Autodesk Inventor part; units mm, degrees
ref_plane "YZ Plane" through (0, 0, 0) normal (1, 0, 0) x (0, 1, 0)
ref_plane "XZ Plane" through (0, 0, 0) normal (0, 1, 0) x (-1, 0, 0)
ref_plane "XY Plane" through (0, 0, 0) normal (0, 0, 1) x (1, 0, 0)
sketch "스케치1" plane through (0, 0, 0) normal (0, 1, 0) x (-1, 0, 0)
  line L0 (23.5, -7) -> (-23.5, -7) construction
  line L1 (-23.5, -7) -> (-23.5, 7) construction
  line L2 (-23.5, 7) -> (23.5, 7) construction
  line L3 (23.5, 7) -> (23.5, -7) construction
  circle A0 centre (23.5, -7) radius 2.1
  circle A1 centre (-23.5, 7) radius 2.1
  circle A2 centre (0, -20) radius 2.1
  circle A3 centre (0, 20) radius 2.1
  circle A4 centre (0, 0) radius 4.5
  circle A5 centre (8, 0) radius 1.6
  circle A6 centre (0, 9.5) radius 1.6
  circle A7 centre (-8, 0) radius 1.6
  circle A8 centre (0, -9.5) radius 1.6
  line L4 (8, 0) -> (0, -9.5) construction
  line L5 (0, -9.5) -> (-8, 0) construction
  line L6 (-8, 0) -> (0, 9.5) construction
  line L7 (0, 9.5) -> (8, 0) construction
  line L8 (10, -10) -> (17, -17) construction
  line L9 (8.8686, -11.1314) -> (15.8686, -18.1314)
  line L10 (18.1314, -15.8686) -> (11.1314, -8.8686)
  arc A9 (11.1314, -8.8686) -> (8.8686, -11.1314) centre (10, -10) ccw
  arc A10 (15.8686, -18.1314) -> (18.1314, -15.8686) centre (17, -17) ccw
  line L11 (-10, -10) -> (-17, -17) construction
  line L12 (-11.1314, -8.8686) -> (-18.1314, -15.8686)
  line L13 (-15.8686, -18.1314) -> (-8.8686, -11.1314)
  arc A11 (-8.8686, -11.1314) -> (-11.1314, -8.8686) centre (-10, -10) ccw
  arc A12 (-18.1314, -15.8686) -> (-15.8686, -18.1314) centre (-17, -17) ccw
  line L14 (10, 10) -> (17, 17) construction
  line L15 (11.1314, 8.8686) -> (18.1314, 15.8686)
  line L16 (15.8686, 18.1314) -> (8.8686, 11.1314)
  arc A13 (8.8686, 11.1314) -> (11.1314, 8.8686) centre (10, 10) ccw
  arc A14 (18.1314, 15.8686) -> (15.8686, 18.1314) centre (17, 17) ccw
  line L17 (-10, 10) -> (-17, 17) construction
  line L18 (-8.8686, 11.1314) -> (-15.8686, 18.1314)
  line L19 (-18.1314, 15.8686) -> (-11.1314, 8.8686)
  arc A15 (-11.1314, 8.8686) -> (-8.8686, 11.1314) centre (-10, 10) ccw
  arc A16 (-15.8686, 18.1314) -> (-18.1314, 15.8686) centre (-17, 17) ccw
  line L20 (10, -10) -> (-10, -10) construction
  line L21 (-10, -10) -> (-10, 10) construction
  line L22 (-10, 10) -> (10, 10) construction
  line L23 (10, 10) -> (10, -10) construction
  circle A17 centre (0, 0) radius 30
  line L24 (42, 0) -> (-42, 0)
  line L25 (0, -42) -> (0, 42)
  line L26 (0, 9.5) -> (0, -9.5) construction
  line L27 (8, 0) -> (-8, 0) construction
  line L28 (28.5, -25) -> (-28.5, -25)
  line L29 (-28.5, -25) -> (-28.5, 25)
  line L30 (-28.5, 25) -> (28.5, 25)
  line L31 (28.5, 25) -> (28.5, -25)
  point P0 (13.5, -13.5)
  point P1 (-13.5, -13.5)
  point P2 (13.5, 13.5)
  point P3 (-13.5, 13.5)
  dimension "d0" = 4.2
  dimension "d1" = 40
  dimension "d2" = 47
  dimension "d3" = 14
  dimension "d4" = 3.2
  dimension "d5" = 16
  dimension "d6" = 19
  dimension "d7" = 9
  dimension "d8" = 20
  dimension "d9" = 34
  dimension "d10" = 1.6
  dimension "d11" = 60
  dimension "d18" = 5
  dimension "d19" = 5
extrude "돌출1" add sketch "스케치1" along normal blind 5 contours A2 L25 A8 A4 L24 A5 L31 A17 L28 | A2 L25 L28 A17 L29 L24 A7 A4 A8 | L28 A17 L25 | L25 A17 L28 | L31 L24 A17 | A17 L24 L29 | L24 A7 L29 A17 L30 L25 A3 A6 A4 | A4 L25 A6 A3 L30 A17 L31 L24 A5 | L24 L31 A17 | A17 L29 L24 | L30 L25 A17 | A17 L25 L30
sketch "스케치2" plane through (0, 0, 0) normal (0, -1, 0) x (1, 0, 0)
  circle A0 centre (0, 0) radius 30
  circle A1 centre (0, 0) radius 4.5
  circle A2 centre (8, 0) radius 1.6
  circle A3 centre (0, -20) radius 2.1
  circle A4 centre (0, -9.5) radius 1.6
  circle A5 centre (-8, 0) radius 1.6
  arc A6 (8.8686, 11.1314) -> (11.1314, 8.8686) centre (10, 10) ccw
  line L0 (15.8686, 18.1314) -> (8.8686, 11.1314)
  arc A7 (18.1314, 15.8686) -> (15.8686, 18.1314) centre (17, 17) ccw
  line L1 (11.1314, 8.8686) -> (18.1314, 15.8686)
  circle A8 centre (23.5, 7) radius 2.1
  arc A9 (-11.1314, 8.8686) -> (-8.8686, 11.1314) centre (-10, 10) ccw
  line L2 (-18.1314, 15.8686) -> (-11.1314, 8.8686)
  arc A10 (-15.8686, 18.1314) -> (-18.1314, 15.8686) centre (-17, 17) ccw
  line L3 (-8.8686, 11.1314) -> (-15.8686, 18.1314)
  circle A11 centre (0, 20) radius 2.1
  circle A12 centre (0, 9.5) radius 1.6
  circle A13 centre (-23.5, -7) radius 2.1
  arc A14 (-8.8686, -11.1314) -> (-11.1314, -8.8686) centre (-10, -10) ccw
  line L4 (-15.8686, -18.1314) -> (-8.8686, -11.1314)
  arc A15 (-18.1314, -15.8686) -> (-15.8686, -18.1314) centre (-17, -17) ccw
  line L5 (-11.1314, -8.8686) -> (-18.1314, -15.8686)
  arc A16 (11.1314, -8.8686) -> (8.8686, -11.1314) centre (10, -10) ccw
  line L6 (18.1314, -15.8686) -> (11.1314, -8.8686)
  arc A17 (15.8686, -18.1314) -> (18.1314, -15.8686) centre (17, -17) ccw
  line L7 (8.8686, -11.1314) -> (15.8686, -18.1314)
  circle A18 centre (0, 20) radius 5
  circle A19 centre (23.5, 7) radius 2.1
  circle A20 centre (23.5, 7) radius 5
  circle A21 centre (0, -20) radius 2.1
  circle A22 centre (0, -20) radius 5
  circle A23 centre (-23.5, -7) radius 2.1
  circle A24 centre (-23.5, -7) radius 5
  dimension "d14" = 10
extrude "돌출2" add sketch "스케치2" along normal blind 3 contours A18 | A20 | A22 | A24
fillet "모깎기1" radius 3 4 edges at (-5, 0, 20) (-28.5, 0, -7) (-5, 0, -20) (18.5, 0, 7)
properties part number "motor_mount" material "PC/ABS 플라스틱"
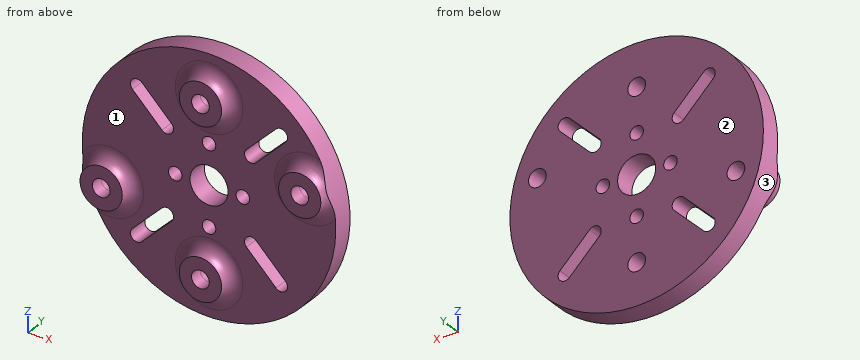
Could you check a few things on this model? Use its own coordinates, in mm. Face numbers are marked on the shaded views. Round coordinates to 2 decimals unless told otherwise and drop trailing zeros. Write each loop counter-clockwise with the first axis right and the second up, starting at its lowest first coordinate (ties: lowest second). Pieces come first, ordered by that corner, then holes. Notation, with made-up numbers: M -36,54.5 L 7,54.5 A26 ccw 7,81.5 Z; hole C 71,16 d5. An arc over 180 degrees is marked long. Answer in a Markdown table with one row per item. Add a question column.
Q1. Imagine slicing it at D-D (x = 14). Please give me the cut outline in (y, z).
Q2. If we mould it in two halves opening along Z, with no side actions, what happens to the marked faces 1, 2 and 3? For each: +Z half, -Z half, draft (parallel to the pull), parting line (faces both ways), or undercut.
Q3. Imagine slicing it at B-B (z = -7). Please give me the cut outline in (x, y).
Q4. Imagine slicing it at C-C (x = -23.5). Please give me the cut outline in (y, z).
Q5. If I drill on line 1 (X direction, y = 1.85, z = 0); line 2 (Z direction, x = 0, y = 1.05); line 3 (X direction, y = 1, z = 11.5), over which ranges is the centre line in solid material (lowest first)? Write a range as from..to.
Q6. Will these pins go through, and if not, where does the flat tip stop? pin 1 Ø5 at (x, z) = (0, -9.5) entering from -Y; pin 2 Ø2 at (y, z) = (0, 9) entering from -X; pin 3 Ø1 at (x, y) = (12.5, 3) entering from -Z; pin 4 Ø5.5 at (x, z) = (0, -20) entering from +Y.
Q7. Imagine slicing it at A-A (y = 2.5). Give the number of separate pieces and of enclosed holes in the cut face, then the cut area to 3 significant figures.
Values:
| question | item | result |
|---|---|---|
| 1 | outline | M 0,-26.53 L 5,-26.53 L 5,-16.26 L 0,-16.26 Z; M 0,-11.74 L 5,-11.74 L 5,11.74 L 0,11.74 Z; M 0,16.26 L 5,16.26 L 5,26.53 L 0,26.53 Z |
| 2 | face 1 | undercut |
| 2 | face 2 | draft |
| 2 | face 3 | parting line |
| 3 | outline | M -29.17,-1.11 A3 cw -28.5,-3 L -25.6,-3 L -25.6,5 L -29.17,5 Z; M -21.4,-3 L -18.5,-3 A3 cw -15.5,0 L 29.17,0 L 29.17,5 L -21.4,5 Z |
| 4 | outline | M -3,-12 A3 cw 0,-15 L 0,-18.65 L 5,-18.65 L 5,-9.1 L -3,-9.1 Z; M -3,-4.9 L 5,-4.9 L 5,18.65 L 0,18.65 L 0,1 A3 cw -3,-2 Z |
| 5 | line 1 | -30..-9.6, -6.4..-4.5, 4.5..6.4, 9.6..30 |
| 5 | line 2 | -30..-22.1, -17.9..-11.1, -7.9..-4.5, 4.5..7.9, 11.1..17.9, 22.1..30 |
| 5 | line 3 | -27.71..-13.76, -9.24..9.24, 13.76..27.71 |
| 6 | pin 1 | y = 0 |
| 6 | pin 2 | x = -28.91 |
| 6 | pin 3 | z = -27.5 |
| 6 | pin 4 | y = 5 |
| 7 | separate pieces | 1 |
| 7 | enclosed holes | 13 |
| 7 | area | 2,520 mm^2 |
